Part model, mm, in its own coordinate system. Give positions to 0.01 mm unless a question says otherwise; leave off trailing zeros. Write each loop counter-clockwise with the first axis right and the second up, starting at its lowest first coordinate (ties: lowest second). Pieces come first, ordered by that corner, then holes. Notation, with made-up numbers: (45, 25) - (65, 25) arc R19 ccw to (65, 40) - close; hole circle Ø7 at (-16, 18.25). An arc over 180 degrees is marked (long way). Answer in a Markdown table with one row per item. Add a question column.
1. Band-saw the part on A-A on x = -70. Write the cut outline in (y, z).
2. Band-saw the part on B-B on y = 30. Write the cut outline in (x, z).
3. Probe line 1 along Y through (x, z) = (-107, -0.5); line 2 along X through (y, z) = (34.5, 0.55); line 3 along X through (y, z) = (41, -0.2). List the from-to ranges inside material, lowest first.
4. Drop a flat-ended pin along its axis: pin 1 Ø20 at (x, y) = (0, 30) entering from -Z (3 decimals). Give the stop position or say it passes through.
5. Band-saw the part on C-C on z = -0.3. State how many separate pieces and enclosed holes the cut face has, plus the area to 3 significant figures.
Autodesk Inventor part; units mm, degrees
ref_plane "YZ Plane" through (0, 0, 0) normal (1, 0, 0) x (0, 1, 0)
ref_plane "XZ Plane" through (0, 0, 0) normal (0, 1, 0) x (-1, 0, 0)
ref_plane "XY Plane" through (0, 0, 0) normal (0, 0, 1) x (1, 0, 0)
sketch "スケッチ1" plane through (0, 0, 0) normal (0, 1, 0) x (-1, 0, 0)
  line L0 (130, 1.5) -> (-130, 1.5)
  line L1 (-130, 1.5) -> (-130, -1.5)
  line L2 (-130, -1.5) -> (130, -1.5)
  line L3 (130, -1.5) -> (130, 1.5)
  line L4 (130, 1.5) -> (-130, -1.5) construction
  line L5 (-130, 1.5) -> (130, -1.5) construction
  point P0 (0, 0)
  dimension "d0" = 260
  dimension "d1" = 3
extrude "押し出し1" add sketch "スケッチ1" along normal blind 60
sketch "スケッチ3" plane through (-130, 0, 1.5) normal (0, 0, 1) x (1, 0, 0)
  circle A0 centre (60, 30) radius 12.5
  circle A1 centre (130, 30) radius 12.5
  circle A2 centre (200, 30) radius 12.5
  line L0 (0, 0) -> (0, 60)
  line L1 (260, 0) -> (260, 60)
  point P0 (130, 0)
  point P1 (0, 30)
  point P2 (260, 30)
  dimension "d10" = 25
  dimension "d11" = 25
  dimension "d12" = 25
  dimension "d15" = 60
  dimension "d16" = 60
  dimension "d18" = 0
  dimension "d21" = 0
extrude "押し出し3" cut sketch "スケッチ3" against normal through all
sketch "スケッチ5" plane through (130, 0, -1.5) normal (0, 0, -1) x (-1, 0, 0)
  line L0 (0, 0) -> (260, 0)
  line L1 (0, 60) -> (3, 60)
  line L2 (3, 60) -> (3, 0)
  line L3 (3, 0) -> (0, 0)
  line L4 (0, 0) -> (0, 60)
  line L5 (0, 45) -> (3, 45)
  line L6 (3, 45) -> (3, 15)
  line L7 (3, 15) -> (0, 15)
  line L8 (0, 15) -> (0, 45)
  line L9 (0, 60) -> (260, 60)
  line L10 (130, 60) -> (130, 0)
  line L11 (260, 0) -> (0, 0)
  line L12 (260, 60) -> (257, 60)
  line L13 (257, 60) -> (257, 0)
  line L14 (260, 0) -> (260, 60)
  line L15 (260, 45) -> (257, 45)
  line L16 (257, 15) -> (260, 15)
  point P0 (1.5, 45)
  point P1 (1.5, 60)
  point P2 (1.5, 15)
  point P3 (1.5, 0)
  point P4 (258.5, 15)
  point P5 (257, 0)
  point P6 (257, 60)
  point P7 (0, 15)
  point P8 (3, 45)
  dimension "d22" = 3
  dimension "d23" = 15
  dimension "d24" = 15
extrude "押し出し4" cut sketch "スケッチ5" against normal through all contours L4 L7 L2 L0 | L4 L5 L2 L7 | L4 L1 L2 L5 | L13 L16 L14 L0 | L13 L15 L14 L16 | L9 L14 L15 L13
sketch "スケッチ8" plane through (-127, 0, 1.5) normal (0, 0, 1) x (1, 0, 0)
  circle A0 centre (20, 50) radius 1.6
  circle A1 centre (20, 10) radius 1.6
  line L0 (0, 60) -> (0, 0)
  line L1 (0, 60) -> (254, 60)
  line L2 (0, 0) -> (254, 0)
  line L3 (127, 60) -> (127, 0)
  circle A2 centre (234, 50) radius 1.6
  circle A3 centre (234, 10) radius 1.6
  dimension "d31" = 20
  dimension "d32" = 10
  dimension "d33" = 20
  dimension "d34" = 10
  dimension "d35" = 3.2
  dimension "d36" = 3.2
extrude "押し出し7" cut sketch "スケッチ8" against normal through all contours A0 | A1 | A2 | A3
fillet "フィレット1" radius 5 4 edges at (-127, 60, 0) (-127, 0, 0) (127, 60, 0) (127, 0, 0)
sketch "スケッチ13" plane through (-122, 0, 1.5) normal (0, 0, 1) x (1, 0, 0)
  line L0 (244, 60) -> (0, 60)
  line L1 (122, 60) -> (122, 0)
  circle A0 centre (15, 50) radius 1.6
  circle A1 centre (15, 10) radius 1.6
  point P0 (26, 50)
  point P1 (26, 10)
  point P2 (218, 50)
  point P3 (218, 10)
  dimension "d60" = 11
  dimension "d61" = 11
  dimension "d62" = 40
  dimension "d63" = 10
hole "穴1" at (-96, 50, 1.5) at (-96, 10, 1.5) at (96, 50, 1.5) at (96, 10, 1.5) direction (0, 0, -1) diameter 3.2 end through all
equation "\"d36\" = d35"
properties part number "BP_BOX-Front-60" material "アセタール樹脂、白"
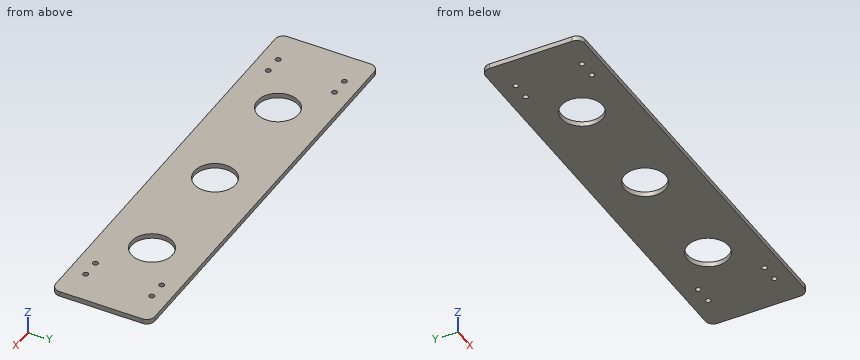
Values:
| question | item | result |
|---|---|---|
| 1 | outline | (0, -1.5) - (17.5, -1.5) - (17.5, 1.5) - (0, 1.5) - close; (42.5, -1.5) - (60, -1.5) - (60, 1.5) - (42.5, 1.5) - close |
| 2 | outline | (-127, -1.5) - (-82.5, -1.5) - (-82.5, 1.5) - (-127, 1.5) - close; (-57.5, -1.5) - (-12.5, -1.5) - (-12.5, 1.5) - (-57.5, 1.5) - close; (12.5, -1.5) - (57.5, -1.5) - (57.5, 1.5) - (12.5, 1.5) - close; (82.5, -1.5) - (127, -1.5) - (127, 1.5) - (82.5, 1.5) - close |
| 3 | line 1 | y = 0 to 8.4, 11.6 to 48.4, 51.6 to 60 |
| 3 | line 2 | x = -127 to -81.66, -58.34 to -11.66, 11.66 to 58.34, 81.66 to 127 |
| 3 | line 3 | x = -127 to -75.94, -64.06 to -5.94, 5.94 to 64.06, 75.94 to 127 |
| 4 | pin 1 | passes through |
| 5 | separate pieces | 1 |
| 5 | enclosed holes | 11 |
| 5 | area | 13,700 mm² |
